```python
from build123d import *

# Parameters (mm, degrees)
BOSS_EXTRUDE1_DEPTH = 668
FILLET1_R           = 1.5


with BuildPart() as part:
    # Sketch1 → Boss-Extrude1 (new body)
    with BuildSketch(Plane.XY):
        with BuildLine():
            Line((-1, 0), (-35, 0))
            Line((-35, 0), (-35, 3))
            Line((-35, 3), (-6, 3))
            ThreePointArc((-6, 3), (-3.878679656, 3.878679656), (-3, 6))
            Line((-3, 6), (-3, 35))
            Line((-3, 35), (0, 35))
            Line((0, 35), (0, 1))
            ThreePointArc((0, 1), (-0.292893219, 0.292893219), (-1, 0))
        make_face()
    extrude(amount=BOSS_EXTRUDE1_DEPTH)

    # Fillet1
    fillet1_edges = [part.edges().sort_by_distance(p)[0] for p in [
        (-35, 3, 334),
        (-3, 35, 334),
    ]]
    fillet(fillet1_edges, radius=FILLET1_R)

    # Mirror4: part across plane


with BuildPart() as part_1:
    add(part.part)
    add(part.part.mirror(Plane.XY))


solid = part_1.part
```
Check sheet for the modelled part. Datum: model origin and axes. Units: mm. A direction names the side the tool comes from. Round coordinates to 2 decimals unless told otherwise and drop trailing zeros. Order: outer loops, then holes, each group sorted by start corner. A loop starts at its lowest first (then second) coordinate and runs counter-clockwise, first axis right, second up. Notation, with made-up numbers: (31, 51.5) -> (88, 51.5) arc R18 ccw to (88, 73.5) -> close; hole circle Ø10 at (-28, 28.25). An arc over 180 degrees is marked (long way). One line per item, written item: value. Start each with the question number.
Q1. Set-up check for faces 1 (the face through (-20, 3, 9)), 2 (the face through (-18, 0, 9)): record each of +Z, -Z, +X, -X, +Y, -Y from which the full face is reachable in a straight line by a thin tool's end or side.
Q2. Gauge pin test, flat ends, axial feed: pin 1 Ø2 at (y, z) = (23.5, 25.5) entering from -X; pin 2 Ø3 at (x, z) = (-19, 253) entering from +Y. Record the tip position at first contact, or that the pin passes through.
Q3. Cross-section at B-B (y = 13). Record the boundary of the cut face in (x, z), and give its area (3 significant figures).
Q4. Cross-section at C-C (x = -22). Record the boundary of the cut face in (y, z), and give its area (3 significant figures).
Q5. Thickness scan on line 1 (Y direction, x = -17, z = -162.5); line 2 (X direction, y = 16, z = -84); line 3 (X direction, y = 2.5, z = 399.5). Record the ranges inside material, lowest first.
Q6. Cross-section at A-A (z = -183). Record the boundary of the cut face in (x, y), and give its area (3 significant figures).
Completed:
1. face 1: +Z, -Z, -X, +Y
1. face 2: +Z, -Z, +X, -X, -Y
2. pin 1: stops at x = -3
2. pin 2: stops at y = 3
3. outline: (-3, -668) -> (0, -668) -> (0, 668) -> (-3, 668) -> close
3. area: 4,010 mm²
4. outline: (0, -668) -> (3, -668) -> (3, 668) -> (0, 668) -> close
4. area: 4,010 mm²
5. line 1: y = 0 to 3
5. line 2: x = -3 to 0
5. line 3: x = -34.62 to 0
6. outline: (-35, 0) -> (-1, 0) arc R1 ccw to (0, 1) -> (0, 35) -> (-1.5, 35) arc R1.5 ccw to (-3, 33.5) -> (-3, 6) arc R3 cw to (-6, 3) -> (-33.5, 3) arc R1.5 ccw to (-35, 1.5) -> close
6. area: 202 mm²
